Here's how the part is built. I have some questions about the finished solid (model axes, mm). A direction names the side the tool comes from. Coordinates: 2 decimals unless noted, no trailing zeros. Loops run counter-clockwise (first coordinate to the right, second up) from the corner with the lowest first, then second, coordinate; pieces in that order, holes last.
Autodesk Inventor part; units mm, degrees
ref_plane "YZ Plane" through (0, 0, 0) normal (1, 0, 0) x (0, 1, 0)
ref_plane "XZ Plane" through (0, 0, 0) normal (0, 1, 0) x (-1, 0, 0)
ref_plane "XY Plane" through (0, 0, 0) normal (0, 0, 1) x (1, 0, 0)
sketch "Sketch1" plane through (0, 0, 0) normal (0, 1, 0) x (-1, 0, 0)
  circle A0 centre (0, 0) radius 30
  circle A1 centre (0, 0) radius 39
  dimension "d0" = 60
  dimension "d1" = 78
extrude "Extrusion1" add sketch "Sketch1" along normal blind 10
sketch "Sketch2" plane through (0, 10, 0) normal (0, 1, 0) x (1, 0, 0)
  circle A0 centre (0, 0) radius 32.5
  circle A1 centre (0, 0) radius 36.5
  dimension "d4" = 65
  dimension "d5" = 73
extrude "Extrusion2" cut sketch "Sketch2" against normal blind 0.7
sketch "Sketch3" plane through (0, 0, 0) normal (0, -1, 0) x (1, 0, 0)
  circle A0 centre (0, 0) radius 36.5
  circle A1 centre (0, 0) radius 32.5
extrude "Extrusion3" cut sketch "Sketch3" against normal blind 0.7
properties part number "bearing_.6812zzipt"
1. On a 3-axis mill with a long thin cutter (end or side, diameter ignored), from which of +Z, -Z, +X, -X, +Y, -Y can I reach the whole of each face in a straight line? I mean faces 1 (the flat face through (-9, 0, -29)), 2 (the flat face through (-33, 0.7, -3)), 3 (the flat face through (-33, 9.3, 3)). Say none if no direction works.
2. I need wall thicknesses on line 1 along Z through (x, y) = (0, 9.5); line 2 along X through (y, z) = (0.5, -22); line 3 along Y through (x, z) = (-12, -32.5). Which ranges of each line are inside material? Lowest first, please.
3. For pin 1 (3 mm diameter, centred on x = 9.5, y = 2, fed in from -Z); pin 2 (1 mm diameter, centred on x = 15, y = 4.5, fed in from +Z); pin 3 (4 mm diameter, centred on x = 5.5, y = 4, fed in from -Z), each with a flat end and sliding along its axis, tell me the tip position at first contact or that it passes through.
4. I want a section at A-A (x = 0). Please give me the cut outline in (y, z).
5. I want a section at C-C (y = 2.75). Please give me the cut outline in (x, z), then the cut area to 3 significant figures.
6. I want a section at B-B (z = 0). Please give me the cut outline in (x, y), then the cut area to 3 significant figures.
7. I want a section at D-D (z = 31). Please give me the cut outline in (x, y).
8. We'd pull the mould along Z, two halves only. Please class faces 4 (the cylindrical face through (-7.912, 9.655, 35.632)), 5 (the cylindrical face through (5.077, 4.93, -38.668)), 6 (the flat face through (-9, 10, -29)): +Z half, -Z half, draft (parallel to the pull), parting line (faces both ways), or undercut.
Response values:
1. face 1: +Z, -Z, +X, -X, -Y
1. face 2: -Y
1. face 3: +Y
2. line 1: z = -39 to -36.5, -32.5 to -30, 30 to 32.5, 36.5 to 39
2. line 2: x = -32.2 to -29.12, -23.92 to -20.4, 20.4 to 23.92, 29.12 to 32.2
2. line 3: y = 0.7 to 9.3
3. pin 1: stops at z = -38.17
3. pin 2: stops at z = 36.2
3. pin 3: stops at z = -38.84
4. outline: (0, -39) - (10, -39) - (10, -36.5) - (9.3, -36.5) - (9.3, -32.5) - (10, -32.5) - (10, -30) - (0, -30) - (0, -32.5) - (0.7, -32.5) - (0.7, -36.5) - (0, -36.5) - close; (0, 30) - (10, 30) - (10, 32.5) - (9.3, 32.5) - (9.3, 36.5) - (10, 36.5) - (10, 39) - (0, 39) - (0, 36.5) - (0.7, 36.5) - (0.7, 32.5) - (0, 32.5) - close
5. outline: circle Ø78 at (0, 0); hole circle Ø60 at (0, 0)
5. area: 1,950 mm2
6. outline: (-39, 0) - (-36.5, 0) - (-36.5, 0.7) - (-32.5, 0.7) - (-32.5, 0) - (-30, 0) - (-30, 10) - (-32.5, 10) - (-32.5, 9.3) - (-36.5, 9.3) - (-36.5, 10) - (-39, 10) - close; (30, 0) - (32.5, 0) - (32.5, 0.7) - (36.5, 0.7) - (36.5, 0) - (39, 0) - (39, 10) - (36.5, 10) - (36.5, 9.3) - (32.5, 9.3) - (32.5, 10) - (30, 10) - close
6. area: 169 mm2
7. outline: (-23.66, 0) - (-19.27, 0) - (-19.27, 0.7) - (-9.76, 0.7) - (-9.76, 0) - (9.76, 0) - (9.76, 0.7) - (19.27, 0.7) - (19.27, 0) - (23.66, 0) - (23.66, 10) - (19.27, 10) - (19.27, 9.3) - (9.76, 9.3) - (9.76, 10) - (-9.76, 10) - (-9.76, 9.3) - (-19.27, 9.3) - (-19.27, 10) - (-23.66, 10) - close
8. face 4: undercut
8. face 5: parting line
8. face 6: draft
